```python
from build123d import *

# Parameters (mm, degrees)
F1_DEPTH = 4
F2_R     = 2.5
F3_DEPTH = 4.001


with BuildPart() as f1:
    # F0 (on Top) → F1 (new body)
    with BuildSketch(Plane.XY):
        with BuildLine():
            ThreePointArc((8.187836, -5.741023), (9.536204, -3.01012), (10, 0))
            ThreePointArc((10, 0), (9.966926, 0.812645), (9.867922, 1.619914))
            ThreePointArc((9.867922, 1.619914), (9.749279, 2.225209), (9.593545, 2.822039))
            ThreePointArc((9.593545, 2.822039), (7.818315, 6.234898), (4.886049, 8.725052))
            ThreePointArc((4.886049, 8.725052), (4.338837, 9.009689), (3.775119, 9.260047))
            ThreePointArc((3.775119, 9.260047), (0, 10), (-3.775119, 9.260047))
            ThreePointArc((-3.775119, 9.260047), (-4.338837, 9.009689), (-4.886049, 8.725052))
            ThreePointArc((-4.886049, 8.725052), (-7.818315, 6.234898), (-9.593545, 2.822039))
            ThreePointArc((-9.593545, 2.822039), (-9.749279, 2.225209), (-9.867922, 1.619914))
            ThreePointArc((-9.867922, 1.619914), (-9.749279, -2.225209), (-8.187836, -5.741023))
            ThreePointArc((-8.187836, -5.741023), (-7.818315, -6.234898), (-7.419048, -6.705052))
            ThreePointArc((-7.419048, -6.705052), (-4.338837, -9.009689), (-0.61652, -9.980977))
            ThreePointArc((-0.61652, -9.980977), (0, -10), (0.61652, -9.980977))
            ThreePointArc((0.61652, -9.980977), (4.338837, -9.009689), (7.419048, -6.705052))
            ThreePointArc((7.419048, -6.705052), (7.818315, -6.234898), (8.187836, -5.741023))
        make_face()
        with BuildLine():
            ThreePointArc((9.867922, 1.619914), (9.966926, 0.812645), (10, 0))
            ThreePointArc((10, 0), (9.536204, -3.01012), (8.187836, -5.741023))
            ThreePointArc((8.187836, -5.741023), (11.228694, -6.113481), (14.178877, -5.28767))
            Line((14.178877, -5.28767), (14.623919, -3.337814))
            Line((14.623919, -3.337814), (15.068961, -1.387958))
            ThreePointArc((15.068961, -1.387958), (12.769244, 0.636109), (9.867922, 1.619914))
        make_face()
        with BuildLine():
            ThreePointArc((4.886049, 8.725052), (7.818315, 6.234898), (9.593545, 2.822039))
            ThreePointArc((9.593545, 2.822039), (11.780688, 4.967253), (12.974452, 7.788684))
            Line((12.974452, 7.788684), (11.727472, 9.352347))
            Line((11.727472, 9.352347), (10.480493, 10.91601))
            ThreePointArc((10.480493, 10.91601), (7.464164, 10.380004), (4.886049, 8.725052))
        make_face()
        with BuildLine():
            ThreePointArc((8.310194, -12.646766), (8.458823, -9.58679), (7.419048, -6.705052))
            ThreePointArc((7.419048, -6.705052), (4.338837, -9.009689), (0.61652, -9.980977))
            ThreePointArc((0.61652, -9.980977), (2.221264, -12.59064), (4.706318, -14.3823))
            Line((4.706318, -14.3823), (6.508256, -13.514533))
            Line((6.508256, -13.514533), (8.310194, -12.646766))
        make_face()
        with BuildLine():
            ThreePointArc((-3.775119, 9.260047), (0, 10), (3.775119, 9.260047))
            ThreePointArc((3.775119, 9.260047), (3.461584, 12.307545), (2, 15))
            Line((2, 15), (0, 15))
            Line((0, 15), (-2, 15))
            ThreePointArc((-2, 15), (-3.461584, 12.307545), (-3.775119, 9.260047))
        make_face()
        with BuildLine():
            ThreePointArc((-4.706318, -14.3823), (-2.221264, -12.59064), (-0.61652, -9.980977))
            ThreePointArc((-0.61652, -9.980977), (-4.338837, -9.009689), (-7.419048, -6.705052))
            ThreePointArc((-7.419048, -6.705052), (-8.458823, -9.58679), (-8.310194, -12.646766))
            Line((-8.310194, -12.646766), (-6.508256, -13.514533))
            Line((-6.508256, -13.514533), (-4.706318, -14.3823))
        make_face()
        with BuildLine():
            ThreePointArc((-9.593545, 2.822039), (-7.818315, 6.234898), (-4.886049, 8.725052))
            ThreePointArc((-4.886049, 8.725052), (-7.464164, 10.380004), (-10.480493, 10.91601))
            Line((-10.480493, 10.91601), (-11.727472, 9.352347))
            Line((-11.727472, 9.352347), (-12.974452, 7.788684))
            ThreePointArc((-12.974452, 7.788684), (-11.780688, 4.967253), (-9.593545, 2.822039))
        make_face()
        with BuildLine():
            ThreePointArc((-14.178877, -5.28767), (-11.228694, -6.113481), (-8.187836, -5.741023))
            ThreePointArc((-8.187836, -5.741023), (-9.749279, -2.225209), (-9.867922, 1.619914))
            ThreePointArc((-9.867922, 1.619914), (-12.769244, 0.636109), (-15.068961, -1.387958))
            Line((-15.068961, -1.387958), (-14.623919, -3.337814))
            Line((-14.623919, -3.337814), (-14.178877, -5.28767))
        make_face()
    extrude(amount=F1_DEPTH)

    # F2 (on face) → F3 (cut, through all)
    with BuildSketch(Plane.XY.offset(4)):
        Circle(F2_R)
    extrude(amount=-F3_DEPTH, mode=Mode.SUBTRACT)


solid = f1.part
```
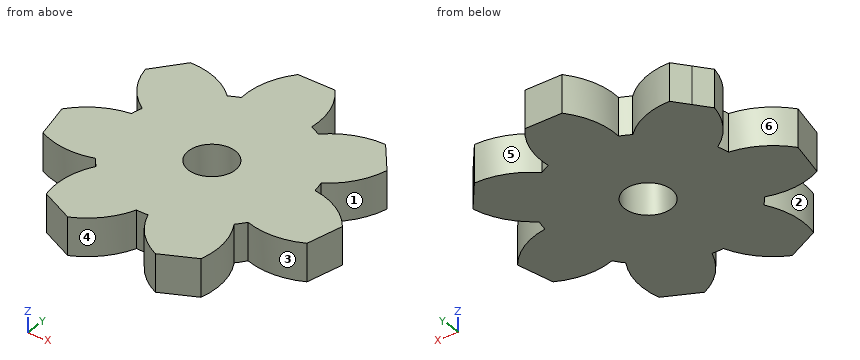
The model under review builds one solid part; all positions refer to its coordinate system, in mm. Face numbers are marked on the shaded views. A direction names the side the tool comes from. Round coordinates to 2 decimals unless told otherwise and drop trailing zeros. Order: outer loops, then holes, each group sorted by start corner. A loop starts at its lowest first (then second) coordinate and runs counter-clockwise, first axis right, second up. Notation, with made-up numbers: (8, 34.5) -> (58, 34.5) arc R32 cw to (58, 66.5) -> close; hole circle Ø6 at (74, 66). An arc over 180 degrees is marked (long way). One line per item, written item: value. Start each with the question number.
Q1. Wall thickness on line 1 (Y direction, x = 0, z = 1.45); line 2 (X direction, y = 9, z = 0.7); line 3 (Y direction, x = -1.5, z = 2): over which ranges is each line inside the solid? List them lowest first.
Q2. Mouldability with a two-part tool opening along X and no side actions: class the marked faces 1, 2 and 3 as released by +X, released by -X, zero draft, split by the parting line, or undercut.
Q3. Take a section at C-C (y = -11.75). Write out the cut boundary in (x, z), and give its area (3 significant figures).
Q4. Machinability: for the marked faces 4, 5 and 6, which of the approach directions +Z, -Z, +X, -X, +Y, -Y give a long, thin tool a straight path to every point of the face, cutting with its end or side? Answer none if there is none.
Q5. Clearance check with flat-ended pins moving along their axes: pin 1 Ø1.5 at (x, z) = (-8, 1) entering from -Y; pin 2 Ø2 at (y, z) = (5, 3.5) entering from -X; pin 3 Ø2 at (x, z) = (3, 0.5) entering from -Y. State where each tip first meets the part, or that it passes through.
Q6. Take a section at B-B (x = 0). Write out the cut boundary in (y, z).
Q7. Take a section at D-D (y = -4). Write out the cut boundary in (x, z).
Reported:
1. line 1: y = -10 to -2.5, 2.5 to 15
1. line 2: x = -12.01 to -5.19, -4.36 to 4.36, 5.19 to 12.01
1. line 3: y = -11.69 to -2, 2 to 15
2. face 1: released by +X
2. face 2: released by -X
2. face 3: undercut
3. outline: (-8.48, 0) -> (-1.54, 0) -> (-1.54, 4) -> (-8.48, 4) -> close; (1.54, 0) -> (8.48, 0) -> (8.48, 4) -> (1.54, 4) -> close
3. area: 55.5 mm2
4. face 4: +Z, -Z, -Y
4. face 5: +Z, -Z, +Y
4. face 6: +Z, -Z, -X
5. pin 1: stops at y = -13.16
5. pin 2: stops at x = -12.37
5. pin 3: stops at y = -14.02
6. outline: (-10, 0) -> (-2.5, 0) -> (-2.5, 4) -> (-10, 4) -> close; (2.5, 0) -> (15, 0) -> (15, 4) -> (2.5, 4) -> close
7. outline: (-14.47, 0) -> (14.47, 0) -> (14.47, 4) -> (-14.47, 4) -> close
